Can you work these out from the model? Positions are in its coordinate system, mm. A direction names the side the tool comes from. Round coordinates to 2 decimals unless told otherwise and drop trailing zeros. Order: outer loops, then holes, each group sorted by start corner. A loop starts at its lowest first (then second) coordinate and runs counter-clockwise, first axis right, second up.
Q1. If I drill on line 1 (Z direction, x = -11.75, y = 12.75); line 2 (Y direction, x = -5, z = 20.5); line 3 (Y direction, x = -5.5, z = 9), over which ranges is the centre line in solid material (lowest first)?
Q2. We'd pull the mould along Z, two halves only. Please class faces 6 (the face through (-5, 12, 0)), 7 (the face through (-5.76, 11.98, 15.87)), 8 (the face through (-13.896, 13.432, 26.876)): pulls with the +Z half, pulls with the -Z half, needs draft (parallel to the pull), parting line crosses it, or undercut.
Q3. Will these pins go through, and if not, where does the flat tip stop? P1, Ø5, axis at x = -8.5, y = 9, coming from the -Z side; P2, Ø6, axis at x = -11.75, z = 6, coming from the -Y side; P3, Ø1, axis at x = -9, z = 17, coming from the -Y side.
Q4. If we section it at B-B (z = 20.5): Please give me the cut outline in (x, y).
Q5. If we section it at C-C (x = -13): Please give me the cut outline in (y, z).
Q6. If we section it at A-A (z = 26.2): Please give me the cut outline in (x, y), plus the area to 3 significant figures.
Q7. For faces 1 (the face through (-5.304, 7.169, 15.875)), 2 (the face through (-13.896, 13.432, 6.676)), 3 (the face through (-14.153, 8.285, 15.875)), 4 (the face through (-11, 16.5, 16)), 5 (the face through (-17, 11.5, 16)), which set-ups out of +Z, -Z, +X, -X, +Y, -Y let a thin tool reach every point of the face, with its end or its side?
Q8. If we section it at D-D (y = 12.5): Please give me the cut outline in (x, z).
from build123d import *

# Parameters (mm, degrees)
F0_R     = 2.1
F1_DEPTH = 32.2
F2_R     = 2.25
F3_DEPTH = 16.501


with BuildPart() as f1:
    # F0 (on Top) → F1 (new body)
    with BuildSketch(Plane.XY):
        with BuildLine():
            Line((-5.7, 16.5), (-15.9, 16.5))
            Line((-15.9, 16.5), (-15.9, 11.5))
            Line((-15.9, 11.5), (-18, 11.5))
            Line((-18, 11.5), (-18, 3.7))
            Line((-18, 3.7), (-10.196373, 13))
            Line((-10.196373, 13), (-6.973896, 13))
            Line((-6.973896, 13), (-4.502056, 10.92588))
            ThreePointArc((-4.502056, 10.92588), (-3.865923, 9.70388), (-4.280194, 8.389982))
            Line((-4.280194, 8.389982), (-6.35776, 5.914035))
            ThreePointArc((-6.35776, 5.914035), (-2.368727, 6.982893), (0, 3.6))
            Line((0, 3.6), (0, 11.717132))
            Line((0, 11.717132), (-5.7, 16.5))
        make_face()
        with BuildLine():
            ThreePointArc((-6.35776, 5.914035), (-4.831273, 0.217107), (0, 3.6))
            ThreePointArc((0, 3.6), (-2.368727, 6.982893), (-6.35776, 5.914035))
        make_face()
        with Locations((-3.6, 3.6)):
            Circle(F0_R, mode=Mode.SUBTRACT)
    extrude(amount=F1_DEPTH)

    # F2 (on face) → F3 (cut, through all)
    with BuildSketch(Plane(origin=(0, 16.5, 0), x_dir=(-1, 0, 0), z_dir=(0, 1, 0))):
        with Locations((11.75, 26.2)):
            Circle(F2_R)
        with Locations((11.75, 6)):
            Circle(F2_R)
    extrude(amount=-F3_DEPTH, mode=Mode.SUBTRACT)


solid = f1.part
Solution:
1. line 1: z = 0 to 3.75, 8.25 to 23.95, 28.45 to 32.2
1. line 2: y = 0.28 to 2.03, 5.17 to 7.53, 11.34 to 15.91
1. line 3: y = 0.54 to 2.71, 4.49 to 6.94, 11.76 to 16.33
2. face 6: pulls with the -Z half
2. face 7: needs draft
2. face 8: undercut
3. P1: passes through
3. P2: stops at y = 7.57
3. P3: stops at y = 13
4. outline: (-18, 3.7) - (-10.2, 13) - (-6.97, 13) - (-4.5, 10.93) arc R1.8 cw to (-4.28, 8.39) - (-6.36, 5.91) arc R3.6 ccw (long way) to (0, 3.6) - (0, 11.72) - (-5.7, 16.5) - (-15.9, 16.5) - (-15.9, 11.5) - (-18, 11.5) - close; hole circle Ø4.2 at (-3.6, 3.6)
5. outline: (9.66, 0) - (16.5, 0) - (16.5, 4.13) - (9.66, 4.13) - close; (9.66, 7.87) - (16.5, 7.87) - (16.5, 24.33) - (9.66, 24.33) - close; (9.66, 28.07) - (16.5, 28.07) - (16.5, 32.2) - (9.66, 32.2) - close
6. outline: (-18, 3.7) - (-14, 8.47) - (-14, 16.5) - (-15.9, 16.5) - (-15.9, 11.5) - (-18, 11.5) - close; (-9.5, 13) - (-6.97, 13) - (-4.5, 10.93) arc R1.8 cw to (-4.28, 8.39) - (-6.36, 5.91) arc R3.6 ccw (long way) to (0, 3.6) - (0, 11.72) - (-5.7, 16.5) - (-9.5, 16.5) - close; hole circle Ø4.2 at (-3.6, 3.6)
6. area: 109 mm2
7. face 1: +Z, -Z
7. face 2: +Y, -Y
7. face 3: +Z, -Z, -Y
7. face 4: +Z, -Z, +X, -X, +Y
7. face 5: +Z, -Z, -X, +Y
8. outline: (-15.9, 0) - (-10.62, 0) - (-10.62, 4.06) arc R2.25 cw (long way) to (-10.62, 7.94) - (-10.62, 24.26) arc R2.25 cw (long way) to (-10.62, 28.14) - (-10.62, 32.2) - (-15.9, 32.2) - close; (-6.38, 0) - (-0.93, 0) - (-0.93, 32.2) - (-6.38, 32.2) - close
